Geometry check sheet. Reference: the model listing, model coordinates, mm. A direction names the side the tool comes from. Round coordinates to 2 decimals unless told otherwise and drop trailing zeros. Loops run counter-clockwise (first coordinate to the right, second up) from the corner with the lowest first, then second, coordinate; pieces in that order, holes last. Notation, with made-up numbers: (-40, 68.5) - (-21, 68.5) arc R25 cw to (-21, 86.5) - close; hole circle Ø11 at (14, 89.25). An arc over 180 degrees is marked (long way). Answer as CSV lines item,"result". Start each with the question number.
1) Access from +Z, -Z, +X, -X, +Y, -Y to the whole of each face (thin tool, end or side, straight path). Record for faces 1 (the flat face through (147, -231, 0)), 2 (the cylindrical face through (-272.786, 12.005, 37.567)).
2) Draft check along X on faces 3 (the cylindrical face through (-0.83, 149.17, 82.46)), 4 (the flat face through (-4, 4, 88.9)), 5 (the cylindrical face through (-285.474, 12.564, 43.828)). Enter one of: released by +X, released by -X, zero draft, split by the parting line, or undercut.
3) Cross-section at A-A on y = 191. Record the boundary of the cut face in (x, z), and give its area (3 significant figures).
4) Thickness scan on line 1 along Y through (x, z) = (0, 81.75) (3 decimals); line 2 along Y through (x, z) = (0, 59.5). Record the ranges inside material, lowest first.
5) Cross-section at B-B on z = 44.5. Record the boundary of the cut face in (x, y), and give its area (3 significant figures).
6) Depth check by flat-ended pin: P1, Ø2, axis at x = 79.5, z = 15, coming from the -Y side; P2, Ø12, axis at y = 68.5, z = 37.5, coming from the -X side; P3, Ø4, axis at x = -0.5, y = 74.5, coming from the -Z side; P4, Ø7.5, axis at x = -142.875, y = 0, coming from the +Z side. Enter the tip coordinate at first touch or a pass-through.
7) Cross-section at C-C on x = 49. Record the boundary of the cut face in (y, z), and give its area (3 significant figures).
from build123d import *

# Parameters (mm, degrees)
F0_R     = 285.75
F0_R_2   = 6.35
F1_DEPTH = 88.9
F2_T     = -12.7
F3_R     = 210.508392
F4_DEPTH = 161.544


with BuildPart() as f1:
    # F0 (on Top) → F1 (new body)
    with BuildSketch(Plane.XY):
        Circle(F0_R)
        with Locations((0, -142.875)):
            Circle(F0_R_2, mode=Mode.SUBTRACT)
        with Locations((-142.875, 0)):
            Circle(F0_R_2, mode=Mode.SUBTRACT)
        with Locations((142.875, 0)):
            Circle(F0_R_2, mode=Mode.SUBTRACT)
        with Locations((0, 142.875)):
            Circle(F0_R_2, mode=Mode.SUBTRACT)
    extrude(amount=F1_DEPTH)

    # F2
    f2_openings = [f1.faces().sort_by_distance(p)[0] for p in [
        (0, 0, 0),
    ]]
    offset(amount=F2_T, openings=f2_openings)

    # F3 (on face) → F4 (cut)
    with BuildSketch(Plane(origin=(0, 0, 76.2), x_dir=(1, 0, 0), z_dir=(0, 0, -1))):
        with Locations((25.252376, -5.049415)):
            Circle(F3_R)
    extrude(amount=F4_DEPTH, mode=Mode.SUBTRACT)


solid = f1.part
Answer block:
1,face 1,"-Z, +X, -X, +Y, -Y"
1,face 2,"-Z"
2,face 3,"undercut"
2,face 4,"zero draft"
2,face 5,"split by the parting line"
3,outline,"(-212.54, 0) - (-195.13, 0) - (-195.13, 76.2) - (195.13, 76.2) - (195.13, 0) - (212.54, 0) - (212.54, 88.9) - (-212.54, 88.9) - close"
3,area,"8,050 mm^2"
4,line 1,"y = -285.75 to -149.225, -136.525 to 136.525, 149.225 to 285.75"
4,line 2,"y = -285.75 to -273.05, 273.05 to 285.75"
5,outline,"circle Ø571.5 at (0, 0); hole circle Ø546.1 at (0, 0)"
5,area,"22,300 mm^2"
6,P1,"stops at y = -274.76"
6,P2,"stops at x = -278.83"
6,P3,"stops at z = 76.2"
6,P4,"passes through"
7,outline,"(-281.52, 0) - (-268.62, 0) - (-268.62, 76.2) - (268.62, 76.2) - (268.62, 0) - (281.52, 0) - (281.52, 88.9) - (-281.52, 88.9) - close"
7,area,"9,120 mm^2"
